The model under review builds one solid part; all positions refer to its coordinate system, in mm. Face numbers are marked on the shaded views. A direction names the side the tool comes from. Round coordinates to 2 decimals unless told otherwise and drop trailing zeros. Write each loop counter-clockwise with the first axis right and the second up, starting at its lowest first coordinate (ties: lowest second). Pieces come first, ordered by that corner, then holes. Notation, with made-up numbers: (5.5, -39) - (50.5, -39) arc R29 ccw to (50.5, -13) - close; hole circle Ø3 at (7.5, 81). An arc over 180 degrees is marked (long way). Return JSON: item names as keys, results as strings.
from build123d import *

# Parameters (mm, degrees)
F1_DEPTH  = 7.5
F2_W      = 7
F2_H      = 2.1077826433
F2_W_2    = 1.5
F2_H_2    = 2.502781529
F2_H_3    = 3.0992894471
F3_DEPTH  = 5
F4_R      = 0.5
F5_DEPTH  = 0.5
F6_R      = 0.5
F7_DEPTH  = 0.5
F8_R      = 0.5
F9_DEPTH  = 0.5
F10_R     = 0.5
F11_DEPTH = 0.5
F13_DEPTH = 4


with BuildPart() as f1:
    # F0 (on Right) → F1 (new body, symmetric)
    with BuildSketch(Plane.YZ):
        with BuildLine():
            ThreePointArc((5, -1), (6, 0), (5, 1))
            Line((5, 1), (-5, 1))
            ThreePointArc((-5, 1), (-6, 0), (-5, -1))
            Line((-5, -1), (5, -1))
        make_face()
    extrude(amount=F1_DEPTH, both=True)

    # F2 (on face) → F3 (cut)
    with BuildSketch(Plane.XY.offset(1)):
        with Locations((0, 5.0538913216)):
            Rectangle(F2_W, F2_H)
        with Locations((-6.75, -5.2513907645)):
            Rectangle(F2_W_2, F2_H_2)
        with Locations((6.75, -5.5496447235)):
            Rectangle(F2_W_2, F2_H_3)
    extrude(amount=-F3_DEPTH, mode=Mode.SUBTRACT)

    # F4 (on face) → F5 (cut)
    with BuildSketch(Plane(origin=(-6, 0, 0), x_dir=(0, -1, 0), z_dir=(-1, 0, 0))):
        with Locations((5, 0)):
            Circle(F4_R)
    extrude(amount=-F5_DEPTH, mode=Mode.SUBTRACT)

    # F6 (on face) → F7 (cut)
    with BuildSketch(Plane.YZ.offset(6)):
        with Locations((-5, 0)):
            Circle(F6_R)
    extrude(amount=-F7_DEPTH, mode=Mode.SUBTRACT)

    # F8 (on face) → F9 (join)
    with BuildSketch(Plane.YZ.offset(-3.5)):
        with Locations((5, 0)):
            Circle(F8_R)
    extrude(amount=F9_DEPTH)

    # F10 (on face) → F11 (join)
    with BuildSketch(Plane(origin=(3.5, 0, 0), x_dir=(0, -1, 0), z_dir=(-1, 0, 0))):
        with Locations((-5, 0)):
            Circle(F10_R)
    extrude(amount=F11_DEPTH)

    # F12 (on Right) → F13 (join, symmetric)
    with BuildSketch(Plane.YZ):
        with BuildLine():
            Line((-2, 1), (2, 1))
            ThreePointArc((2, 1), (0, 3), (-2, 1))
        make_face()
    extrude(amount=F13_DEPTH, both=True)


solid = f1.part
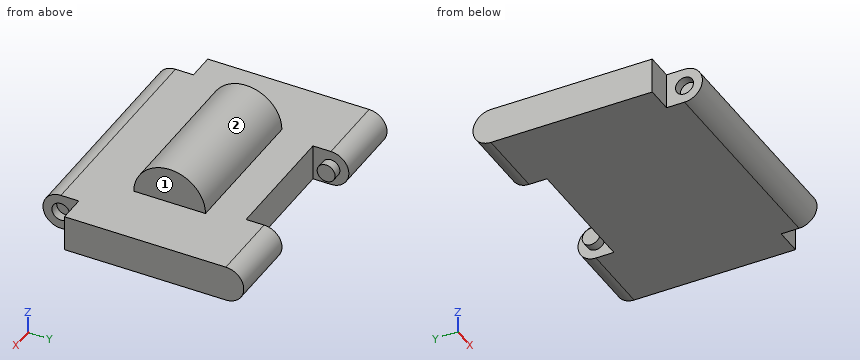
(1) For the marked faces 1 and 2, list the 3-axis set-ups (+Z, -Z, +X, -X, +Y, -Y) from which the entire face can be reached by the end or side of a thin tool; tool diameter is ignored.
Filled in:
{"face 1": "+Z, +X, +Y, -Y", "face 2": "+Z, +X, -X"}
(2) Add section D-D (x = -3.75). Write out the cut boundary in (y, z).
Filled in:
{"outline": "(-5, -1) - (5, -1) arc R1 ccw to (5, 1) - (2, 1) arc R2 ccw to (-2, 1) - (-5, 1) arc R1 ccw to start"}
(3) Wall thickness on line 1 (Z direction, x = 5.75, y = -5); line 2 (Z direction, x = 1.25, y = 3.5); line 3 (X direction, y = 1.25, z = 1.35): over which ranges is each line inside the solid? List them lowest first.
Filled in:
{"line 1": "z = -1 to -0.5, 0.5 to 1", "line 2": "z = -1 to 1", "line 3": "x = -4 to 4"}
(4) Clearance check with flat-ended pins moving along their axes: pin 1 Ø0.6 at (y, z) = (-5, -0.5) entering from -X; pin 2 Ø1.6 at (y, z) = (0.5, 2) entering from +X; pin 3 Ø1.6 at (x, z) = (1, -0.5) entering from +Y. State where each tip first meets the part, or that it passes through.
Filled in:
{"pin 1": "stops at x = -6", "pin 2": "stops at x = 4", "pin 3": "stops at y = 4"}
(5) Add section C-C (z = 0). Write out the cut boundary in (x, y).
Filled in:
{"outline": "(-7.5, -4) - (-6, -4) - (-6, -4.5) - (-5.5, -4.5) - (-5.5, -5.5) - (-6, -5.5) - (-6, -6) - (6, -6) - (6, -5.5) - (5.5, -5.5) - (5.5, -4.5) - (6, -4.5) - (6, -4) - (7.5, -4) - (7.5, 6) - (3.5, 6) - (3.5, 5.5) - (3, 5.5) - (3, 4.5) - (3.5, 4.5) - (3.5, 4) - (-3.5, 4) - (-3.5, 4.5) - (-3, 4.5) - (-3, 5.5) - (-3.5, 5.5) - (-3.5, 6) - (-7.5, 6) - close"}
(6) Add section A-A (y = 0). Write out the cut boundary in (x, z), plus the area to 3 significant figures.
Filled in:
{"outline": "(-7.5, -1) - (7.5, -1) - (7.5, 1) - (4, 1) - (4, 3) - (-4, 3) - (-4, 1) - (-7.5, 1) - close", "area": "46.0 mm2"}
(7) Add section B-B (x = -1.5). Write out the cut boundary in (y, z), plus the area to 3 significant figures.
Filled in:
{"outline": "(-5, -1) - (4, -1) - (4, 1) - (2, 1) arc R2 ccw to (-2, 1) - (-5, 1) arc R1 ccw to start", "area": "25.9 mm2"}
